Verification items for the finished model (mm, model axes). Face numbers are marked on the shaded views. A direction names the side the tool comes from. Give positions to 0.01 mm unless a question says otherwise; leave off trailing zeros. Order: outer loops, then holes, each group sorted by start corner. A loop starts at its lowest first (then second) coordinate and runs counter-clockwise, first axis right, second up. Notation, with made-up numbers: (33, 15.25) -> (56, 15.25) arc R21 ccw to (56, 44.25) -> close; hole circle Ø11 at (73, -26). An arc over 180 degrees is marked (long way). Return JSON: item names as keys, results as strings. Group by question number.
(1) Tool access check on the marked faces 1 and 2. Record the directions out of +Z, -Z, +X, -X, +Y, -Y that give a thin tool (end or side, any length) a straight path to the whole face; none if there is none.
(2) Cross-section at D-D on x = -7.5. Enter the section's corners in (y, z), then the cut area to 3 significant figures.
(3) Thickness scan on line 1 along Z through (x, y) = (-22, 3.45) (3 decimals); line 2 along X through (y, z) = (1.65, -2); line 3 along X through (y, z) = (3, -3). Record the ranges inside material, lowest first.
(4) Cross-section at B-B on x = 31.75. Enter the section's corners in (y, z).
(5) Cross-section at C-C on z = -6.5. Enter the section's corners in (x, y).
(6) Release check for a two-part mould opening along X. For the marked faces 3 and 4 record: pulls with the +X half, pulls with the -X half, needs draft (parallel to the pull), parting line crosses it, or undercut.
(7) Depth check by flat-ended pin: pin 1 Ø2.5 at (x, z) = (38.5, 0) entering from -Y; pin 2 Ø1.2 at (y, z) = (2, 3) entering from +X. Enter the tip coordinate at first touch or a pass-through.
(8) Cross-section at A-A on x = 11.5. Enter the section's corners in (y, z) (3 decimals), then the cut area to 3 significant figures.
from build123d import *

# Parameters (mm, degrees)
EXTRUDE_1_DEPTH     = 4
SKETCH_3_R          = 1.525
CUT_EXTRUDE_2_DEPTH = 5
SKETCH_4_R          = 9
CUT_EXTRUDE_3_DEPTH = 5
CUT_EXTRUDE_4_DEPTH = 5
FILLET_1_R          = 1
FILLET_2_R          = 2
SKETCH_7_R          = 1.525
CUT_EXTRUDE_5_DEPTH = 5


with BuildPart() as part:
    # 草图1 → 凸台-拉伸1 (new body)
    with BuildSketch(Plane(origin=(0, 0, 0), x_dir=(1, 0, 0), z_dir=(0, 1, 0))):
        with BuildLine():
            Line((-25, 17.5), (-25, -17.5))
            Line((-25, -17.5), (25, -17.5))
            ThreePointArc((25, -17.5), (7.5, 0), (25, 17.5))
            Line((25, 17.5), (-25, 17.5))
        make_face()
        with BuildLine():
            ThreePointArc((25, 17.5), (7.5, 0), (25, -17.5))
            Line((25, -17.5), (25, 17.5))
        make_face()
        with BuildLine():
            Line((25, 17.5), (25, -17.5))
            ThreePointArc((25, -17.5), (37.374368671, -12.374368671), (42.5, 0))
            ThreePointArc((42.5, 0), (37.374368671, 12.374368671), (25, 17.5))
        make_face()
    extrude(amount=EXTRUDE_1_DEPTH)

    # 草图3 → 切除-拉伸2 (cut, through all)
    with BuildSketch(Plane(origin=(0, 4, 0), x_dir=(1, 0, 0), z_dir=(0, 1, 0))):
        with Locations((38.5, 0)):
            Circle(SKETCH_3_R)
        with Locations((31.75, -11.691342951)):
            Circle(SKETCH_3_R)
        with Locations((18.25, -11.691342951)):
            Circle(SKETCH_3_R)
        with Locations((11.5, 0)):
            Circle(SKETCH_3_R)
        with Locations((18.25, 11.691342951)):
            Circle(SKETCH_3_R)
        with Locations((31.75, 11.691342951)):
            Circle(SKETCH_3_R)
    extrude(amount=-CUT_EXTRUDE_2_DEPTH, mode=Mode.SUBTRACT)

    # 草图4 → 切除-拉伸3 (cut, through all)
    with BuildSketch(Plane(origin=(0, 4, 0), x_dir=(1, 0, 0), z_dir=(0, 1, 0))):
        with Locations((25, 0)):
            Circle(SKETCH_4_R)
    extrude(amount=-CUT_EXTRUDE_3_DEPTH, mode=Mode.SUBTRACT)

    # 草图5 → 切除-拉伸4 (cut, through all)
    with BuildSketch(Plane(origin=(0, 4, 0), x_dir=(1, 0, 0), z_dir=(0, 1, 0))):
        Polygon((-14.773080244, 13), (-6, 2.631814257), (2.773080244, 13), align=None)
        Polygon((5, 10.67781095), (-3.904075524, 0.154812603), (5, -10.368185743), align=None)
        Polygon((-6, -2.32218905), (-15.035070804, -13), (3.035070804, -13), align=None)
        Polygon((-17, 10.67781095), (-17, -10.368185743), (-8.095924476, 0.154812603), align=None)
    extrude(amount=-CUT_EXTRUDE_4_DEPTH, mode=Mode.SUBTRACT)

    # 圆角1
    fillet_1_edges = [part.edges().sort_by_distance(p)[0] for p in [
        (-15.035070804, 2, 13),
        (-6, 2, 2.32218905),
        (3.035070804, 2, 13),
        (-3.904075524, 2, -0.154812603),
        (5, 2, -10.67781095),
        (5, 2, 10.368185743),
        (-17, 2, 10.368185743),
        (-17, 2, -10.67781095),
        (-8.095924476, 2, -0.154812603),
        (-6, 2, -2.631814257),
        (-14.773080244, 2, -13),
        (2.773080244, 2, -13),
    ]]
    fillet(fillet_1_edges, radius=FILLET_1_R)

    # 圆角2
    fillet_2_edges = [part.edges().sort_by_distance(p)[0] for p in [
        (-25, 2, 17.5),
        (-25, 2, -17.5),
    ]]
    fillet(fillet_2_edges, radius=FILLET_2_R)

    # 草图7 → 切除-拉伸5 (cut, through all)
    with BuildSketch(Plane(origin=(0, 4, 0), x_dir=(1, 0, 0), z_dir=(0, 1, 0))):
        with Locations((-22, 0)):
            Circle(SKETCH_7_R)
        with Locations((-22, 12)):
            Circle(SKETCH_7_R)
        with Locations((-22, -12)):
            Circle(SKETCH_7_R)
    extrude(amount=-CUT_EXTRUDE_5_DEPTH, mode=Mode.SUBTRACT)


solid = part.part
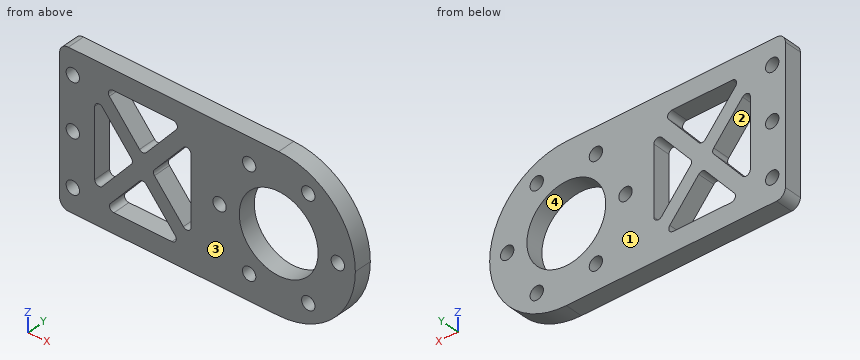
Verdict:
{
 "1": {"face 1": "+Z, -Z, +X, -X, +Y", "face 2": "+Y, -Y"},
 "2": {"outline": "(0, -17.5) -> (4, -17.5) -> (4, -13) -> (0, -13) -> close; (0, -4.4) -> (4, -4.4) -> (4, 4.09) -> (0, 4.09) -> close; (0, 13) -> (4, 13) -> (4, 17.5) -> (0, 17.5) -> close", "area": "70.0 mm²"},
 "3": {"line 1": "-17.5 to -13.525, -10.475 to -1.525, 1.525 to 10.475, 13.525 to 17.5", "line 2": "-25 to -17, -9.66 to -2.34, 5 to 16.23, 33.77 to 42.39", "line 3": "-25 to -17, -10.5 to -1.5, 5 to 16.51, 33.49 to 42.24"},
 "4": {"outline": "(0, -16.15) -> (4, -16.15) -> (4, -13.22) -> (0, -13.22) -> close; (0, -10.17) -> (4, -10.17) -> (4, -5.95) -> (0, -5.95) -> close; (0, 5.95) -> (4, 5.95) -> (4, 10.17) -> (0, 10.17) -> close; (0, 13.22) -> (4, 13.22) -> (4, 16.15) -> (0, 16.15) -> close"},
 "5": {"outline": "(-25, 0) -> (-17, 0) -> (-17, 4) -> (-25, 4) -> close; (-13.46, 0) -> (-9.27, 0) -> (-9.27, 4) -> (-13.46, 4) -> close; (-2.73, 0) -> (1.46, 0) -> (1.46, 4) -> (-2.73, 4) -> close; (5, 0) -> (18.78, 0) -> (18.78, 4) -> (5, 4) -> close; (31.22, 0) -> (41.25, 0) -> (41.25, 4) -> (31.22, 4) -> close"},
 "6": {"face 3": "needs draft", "face 4": "undercut"},
 "7": {"pin 1": "through", "pin 2": "x = 42.33"},
 "8": {"outline": "(0, -17.5) -> (4, -17.5) -> (4, -1.525) -> (0, -1.525) -> close; (0, 1.525) -> (4, 1.525) -> (4, 17.5) -> (0, 17.5) -> close", "area": "128 mm²"}
}
